Model file for the job. Use its own axes, mm. A direction names the side the tool comes from. Round coordinates to 2 decimals unless told otherwise and drop trailing zeros. Loops run counter-clockwise (first coordinate to the right, second up) from the corner with the lowest first, then second, coordinate; pieces in that order, holes last. Notation, with made-up numbers: M -37,60.25 L 18,60.25 A6 ccw 18,70.25 Z; hole C 19,-8 d8. An arc over 180 degrees is marked long. Use a Markdown table: item, result. Add a question column.
Q1. Pin check, flat tips, straight feed: pin 1 (3 mm diameter, centred on y = 68.5, z = 5.5, fed in from +X); pin 2 (2 mm diameter, centred on y = 79.5, z = 1.5, fed in from -X). Stop position of each tip, or through.
Q2. Probe line 1 (X direction, y = -162, z = 5.5) (3 decimals); line 2 (X direction, y = -170, z = 3.15); line 3 (X direction, y = -4, z = 0.3). List the from-to ranges inside material, lowest first. Write a range as from..to.
Q3. Tool access for faces 4 (the face through (88.35, -143.73, 2.96)), 5 (the face through (3, -138, 6)): list every direction of +Z, -Z, +X, -X, +Y, -Y with a clear straight run to the whole face (end or side of a thin tool).
Q4. Cut at B-B (y = -265). Give the cut face in (x, z).
Q5. Cut at A-A (z = 2.05). Give the cut face in (x, y), plus the area to 3 significant figures.
Q6. Mould opens along X. For faces 1 (the face through (2.367, -329.296, 2.958)), 2 (the face through (3, -138, 0)), 3 (the face through (-48.7, -174.4, 3)) say: +X half, -X half, draft (parallel to the pull), parting line (faces both ways), or undercut.
Q7. Cut at C-C (x = 69). Give the cut face in (y, z).
from build123d import *

# Parameters (mm, degrees)
F0_W     = 60
F0_H     = 220
F1_DEPTH = 6


# Not quite as in the source:
# - the program builds the solid bodies; features that only make, move or delete a surface that nothing else refers to are left out


with BuildPart() as f1:
    # F0 (on Top) → F1 (new body)
    with BuildSketch(Plane.XY):
        with Locations((4.8876879096, 45.2179194741)):
            Rectangle(F0_W, F0_H)
        with BuildLine():
            ThreePointArc((-79.4584430704, -175.2136584167), (-76.086405566, -164.9666401832), (-71.4764851469, -155.2136584167))
            ThreePointArc((-71.4764851469, -155.2136584167), (-79.1565485083, -145.3205641479), (-85.5490516624, -134.5505784994))
            ThreePointArc((-85.5490516624, -134.5505784994), (6.1468085688, -329.3233337338), (94.4628409087, -132.9949471034))
            ThreePointArc((94.4628409087, -132.9949471034), (88.2574232589, -143.8738017875), (80.7494829473, -153.8981481364))
            ThreePointArc((80.7494829473, -153.8981481364), (85.2254366965, -162.8589485125), (88.6456429035, -172.2734211397))
            ThreePointArc((88.6456429035, -172.2734211397), (75.2367314586, -249.2062042963), (5.6459887203, -284.6403764396))
            ThreePointArc((5.6459887203, -284.6403764396), (-63.9155377146, -250.9329661403), (-79.4584430704, -175.2136584167))
        make_face()
        with BuildLine():
            ThreePointArc((4.8876879096, -189.3289751767), (-10.6634233248, -188.2490297182), (-25.8614792361, -184.7816907769))
            ThreePointArc((-25.8614792361, -184.7816907769), (-48.9823809676, -174.2243385437), (-68.7229965841, -158.2136584167))
            ThreePointArc((-68.7229965841, -158.2136584167), (-72.9335538665, -167.9839691049), (-75.8560904631, -178.2136584167))
            ThreePointArc((-75.8560904631, -178.2136584167), (-59.2361153237, -247.9542245013), (5.5975931326, -278.5574984969))
            Line((5.5975931326, -278.5574984969), (4.8876879096, -189.3289751767))
        make_face()
        with BuildLine():
            ThreePointArc((78.0917461365, -156.8981481364), (57.9442467877, -173.7054474984), (34.1385207639, -184.7369682609))
            ThreePointArc((34.1385207639, -184.7369682609), (19.6828166371, -188.1140297879), (4.8876879096, -189.3289751767))
            Line((4.8876879096, -189.3289751767), (5.5975931326, -278.5574984969))
            ThreePointArc((5.5975931326, -278.5574984969), (70.4913174106, -246.4384867175), (85.2871903638, -175.5589515052))
            ThreePointArc((85.2871903638, -175.5589515052), (82.255170922, -166.010419768), (78.0917461365, -156.8981481364))
        make_face()
        with BuildLine():
            ThreePointArc((5.5975931326, -278.5574984969), (-59.2361153237, -247.9542245013), (-75.8560904631, -178.2136584167))
            Line((-75.8560904631, -178.2136584167), (-79.4584430704, -175.2136584167))
            ThreePointArc((-79.4584430704, -175.2136584167), (-63.9155377146, -250.9329661403), (5.6459887203, -284.6403764396))
            Line((5.6459887203, -284.6403764396), (5.5975931326, -278.5574984969))
        make_face()
        with BuildLine():
            ThreePointArc((85.2871903638, -175.5589515052), (70.4913174106, -246.4384867175), (5.5975931326, -278.5574984969))
            Line((5.5975931326, -278.5574984969), (5.6459887203, -284.6403764396))
            ThreePointArc((5.6459887203, -284.6403764396), (75.2367314586, -249.2062042963), (88.6456429035, -172.2734211397))
            Line((88.6456429035, -172.2734211397), (85.2871903638, -175.5589515052))
        make_face()
        with BuildLine():
            Line((34.7627821954, -84.7816907769), (-25.2371712536, -84.7816907769))
            Line((-25.2371712536, -84.7816907769), (-25.8614792361, -184.7816907769))
            ThreePointArc((-25.8614792361, -184.7816907769), (-10.6634233248, -188.2490297182), (4.8876879096, -189.3289751767))
            ThreePointArc((4.8876879096, -189.3289751767), (19.6828166371, -188.1140297879), (34.1385207639, -184.7369682609))
            Line((34.1385207639, -184.7369682609), (34.7627821954, -84.7816907769))
        make_face()
        Polygon((34.8876879096, -64.7820805259), (-25.1123120904, -64.7820805259), (-25.2371712536, -84.7816907769), (34.7627821954, -84.7816907769), align=None)
    extrude(amount=F1_DEPTH)


solid = f1.part
Checked values:
| question | item | result |
|---|---|---|
| 1 | pin 1 | stops at x = 34.89 |
| 1 | pin 2 | stops at x = -25.11 |
| 2 | line 1 | x = -102.839..-74.839, -70.533..-64.905, -25.719..34.281, 73.039..80.587, 84.851..113.085 |
| 2 | line 2 | x = -106.11..-77.92, -73.62..-55.26, -25.77..34.23, 63.39..83.68, 87.93..116.36 |
| 2 | line 3 | x = -25.11..34.89 |
| 3 | face 4 | +Z, -Z, +Y |
| 3 | face 5 | +Z, +X, -X, +Y, -Y |
| 4 | outline | M -100.27,0 L 110.51,0 L 110.51,6 L -100.27,6 Z |
| 5 | outline | M -85.55,-134.55 A118.49 ccw long 94.46,-132.99 A100.69 cw 80.75,-153.9 A87.31 cw 88.65,-172.27 L 85.29,-175.56 A82.77 ccw 78.09,-156.9 A100.69 cw 34.14,-184.74 L 34.89,-64.78 L 34.89,155.22 L -25.11,155.22 L -25.11,-64.78 L -25.86,-184.78 A100.69 cw -68.72,-158.21 A82.77 ccw -75.86,-178.21 L -79.46,-175.21 A87.31 cw -71.48,-155.21 A100.69 cw Z |
| 5 | area | 52,200 mm^2 |
| 6 | face 1 | parting line |
| 6 | face 2 | draft |
| 6 | face 3 | undercut |
| 7 | outline | M -310.64,0 L -165.6,0 L -165.6,6 L -310.64,6 Z |
